Source: CAD feature listing. Evaluate the final solid. Frame: model axes, mm. Give positions to 0.01 mm unless a question says otherwise; leave off trailing zeros. Loops run counter-clockwise (first coordinate to the right, second up) from the corner with the lowest first, then second, coordinate; pieces in that order, holes last. Notation, with made-up numbers: (46, 42) -> (55, 42) arc R37 ccw to (55, 79) -> close; hole circle Ø3 at (36.5, 73). An arc over 180 degrees is marked (long way). Return JSON: item names as keys, results as strings. Group by question number.
(1) Ray query, line 1 (X direction, y = 14.8, z = 3.4); line 2 (Y direction, x = 0, z = 3); line 3 (Y direction, x = 17, z = 3.5). Return the intervals inside material, ascending. Write a range as from..to.
(2) Pin query (flat end, axial travel): pin 1 (2.5 mm diameter, centred on x = 15.97, y = 25.41, fed in from -Z); pin 2 (4 mm diameter, centred on x = -15.97, y = 25.41, fed in from -Z); pin 3 (1.5 mm diameter, centred on y = 27, z = 7, fed in from +X). Return the tip coordinate at first contact, or that it passes through.
(3) Cut plane C-C on z = 6.25. Give the number of separate pieces and of enclosed holes in the cut face, then the cut area to 3 significant figures.
(4) Cut plane D-D on x = -29.5. Return loops of the section in (y, z), then the cut area to 3 significant figures.
(5) Cut plane A-A on x = 0. Return loops of the section in (y, z).
(6) Draft query along Y for faces 1 (the face through (33.98, 38.53, 3.94)), 2 (the face through (9, 27, 0)), 3 (the face through (27.64, 17.72, 4.86)). Return one class per face: released by +Y, released by -Y, zero draft, split by the parting line, or undercut.
(7) Cut plane B-B on y = 47.8. Return loops of the section in (x, z), then the cut area to 3 significant figures.
```python
from build123d import *

# Parameters (mm, degrees)
SKETCH_1_R                = 20
SKETCH_1_R_2              = 1.5
SKETCH_1_R_3              = 3
EXTRUDE_1_DEPTH           = 8
HOLE_WIZARD_1_D           = 3.4
HOLE_WIZARD_1_DEPTH       = 8.1
HOLE_WIZARD_1_CSINK_D     = 6.6
HOLE_WIZARD_1_CSINK_ANGLE = 90
HOLE_WIZARD_1_TIP         = 1.021463052
HOLE_WIZARD_2_D           = 6.6
HOLE_WIZARD_2_DEPTH       = 8.1
HOLE_WIZARD_2_CSINK_D     = 13.2
HOLE_WIZARD_2_CSINK_ANGLE = 90
HOLE_WIZARD_2_TIP         = 1.982840043
CHAMFER_1_SIZE            = 1


with BuildPart() as part:
    # 草图1 → 凸台-拉伸1 (new body)
    with BuildSketch(Plane.XY):
        with BuildLine():
            Line((-37.719505087, 14.893838596), (-30.34379321, 61.5147356))
            ThreePointArc((-30.34379321, 61.5147356), (-23.579766095, 73.596472023), (-10.589482469, 78.389482469))
            Line((-10.589482469, 78.389482469), (10.589482469, 78.389482469))
            ThreePointArc((10.589482469, 78.389482469), (23.579766095, 73.596472023), (30.34379321, 61.5147356))
            Line((30.34379321, 61.5147356), (37.719505087, 14.893838596))
            ThreePointArc((37.719505087, 14.893838596), (36.127942671, 9.253400731), (30.805496327, 6.8))
            Line((30.805496327, 6.8), (-30.805496327, 6.8))
            ThreePointArc((-30.805496327, 6.8), (-36.127942671, 9.253400731), (-37.719505087, 14.893838596))
        make_face()
        with Locations((0, 47.8)):
            Circle(SKETCH_1_R, mode=Mode.SUBTRACT)
        with Locations((-15.969331282, 70.188176755)):
            Circle(SKETCH_1_R_2, mode=Mode.SUBTRACT)
        with Locations((-22.388176755, 63.769331282)):
            Circle(SKETCH_1_R_2, mode=Mode.SUBTRACT)
        with Locations((-22.388176755, 31.830668718)):
            Circle(SKETCH_1_R_2, mode=Mode.SUBTRACT)
        with Locations((-15.969331282, 25.411823245)):
            Circle(SKETCH_1_R_2, mode=Mode.SUBTRACT)
        with Locations((15.969331282, 25.411823245)):
            Circle(SKETCH_1_R_2, mode=Mode.SUBTRACT)
        with Locations((22.388176755, 31.830668718)):
            Circle(SKETCH_1_R_2, mode=Mode.SUBTRACT)
        with Locations((22.388176755, 63.769331282)):
            Circle(SKETCH_1_R_2, mode=Mode.SUBTRACT)
        with Locations((15.969331282, 70.188176755)):
            Circle(SKETCH_1_R_2, mode=Mode.SUBTRACT)
        with Locations((-29.5, 14.8)):
            Circle(SKETCH_1_R_3, mode=Mode.SUBTRACT)
        with Locations((0, 14.8)):
            Circle(SKETCH_1_R_3, mode=Mode.SUBTRACT)
        with Locations((29.5, 14.8)):
            Circle(SKETCH_1_R_3, mode=Mode.SUBTRACT)
    extrude(amount=EXTRUDE_1_DEPTH)

    # 打孔尺寸(%根据十字)槽沉头木螺钉的类型1
    with Locations(Plane(origin=(0, 0, 0), x_dir=(-1, 0, 0), z_dir=(0, 0, -1))):
        with Locations((-22.388176755, 63.769331282), (-15.969331282, 70.188176755), (15.969331282, 70.188176755), (22.388176755, 63.769331282), (-22.388176755, 31.830668718), (-15.969331282, 25.411823245), (15.969331282, 25.411823245), (22.388176755, 31.830668718)):
            CounterSinkHole(HOLE_WIZARD_1_D / 2, HOLE_WIZARD_1_CSINK_D / 2, depth=HOLE_WIZARD_1_DEPTH, counter_sink_angle=HOLE_WIZARD_1_CSINK_ANGLE)
            with Locations((0, 0, -(HOLE_WIZARD_1_DEPTH + HOLE_WIZARD_1_TIP / 2))):  # 118° drill point
                Cone(0, HOLE_WIZARD_1_D / 2, HOLE_WIZARD_1_TIP, mode=Mode.SUBTRACT)

    # 打孔尺寸(%根据十字)槽沉头木螺钉的类型2
    with Locations(Plane.XY.offset(8)):
        with Locations((29.5, 14.8), (0, 14.8), (-29.5, 14.8)):
            CounterSinkHole(HOLE_WIZARD_2_D / 2, HOLE_WIZARD_2_CSINK_D / 2, depth=HOLE_WIZARD_2_DEPTH, counter_sink_angle=HOLE_WIZARD_2_CSINK_ANGLE)
            with Locations((0, 0, -(HOLE_WIZARD_2_DEPTH + HOLE_WIZARD_2_TIP / 2))):  # 118° drill point
                Cone(0, HOLE_WIZARD_2_D / 2, HOLE_WIZARD_2_TIP, mode=Mode.SUBTRACT)

    # 倒角1
    chamfer_1_edges = [part.edges().sort_by_distance(p)[0] for p in [
        (-20, 47.8, 0),
    ]]
    chamfer(chamfer_1_edges, length=CHAMFER_1_SIZE)


solid = part.part
```
Answers:
{
 "1": {"line 1": "-37.73..-32.8, -26.2..-3.3, 3.3..26.2, 32.8..37.73", "line 2": "6.8..11.5, 18.1..27.8, 67.8..78.39", "line 3": "6.8..24.06, 26.76..37.26, 58.34..68.84, 71.54..77.33"},
 "2": {"pin 1": "through", "pin 2": "z = 1.3", "pin 3": "x = 35.92"},
 "3": {"separate pieces": "1", "enclosed holes": "12", "area": "3,070 mm²"},
 "4": {"outline": "(6.8, 0) -> (11.5, 0) -> (11.5, 4.7) -> (8.2, 8) -> (6.8, 8) -> close; (18.1, 0) -> (64.9, 0) -> (64.9, 8) -> (21.4, 8) -> (18.1, 4.7) -> close", "area": "401 mm²"},
 "5": {"outline": "(6.8, 0) -> (11.5, 0) -> (11.5, 4.7) -> (8.2, 8) -> (6.8, 8) -> close; (18.1, 0) -> (26.8, 0) -> (27.8, 1) -> (27.8, 8) -> (21.4, 8) -> (18.1, 4.7) -> close; (67.8, 1) -> (68.8, 0) -> (78.39, 0) -> (78.39, 8) -> (67.8, 8) -> close"},
 "6": {"face 1": "released by +Y", "face 2": "zero draft", "face 3": "undercut"},
 "7": {"outline": "(-32.51, 0) -> (-21, 0) -> (-20, 1) -> (-20, 8) -> (-32.51, 8) -> close; (20, 1) -> (21, 0) -> (32.51, 0) -> (32.51, 8) -> (20, 8) -> close", "area": "199 mm²"}
}
